Drawing for the job (mm, zero at the part's lowest x, y, z). A direction names the side the tool comes from. Give positions to 0.01 mm unless a question says otherwise; leave off trailing zeros. Loops run counter-clockwise (first coordinate to the right, second up) from the corner with the lowest first, then second, coordinate; pieces in that order, holes last. Notation, with made-up numbers: (53, 46.25) - (65, 46.25) arc R21 ccw to (65, 72.25) - close; hole circle Ø11 at (13.5, 16). An arc over 180 degrees is marked (long way). Return JSON: item names as keys, results as strings. Group by question number.
1) 3-axis set-ups, long thin cutter, end or side, ignore diameter. For the marked faces 4 and 5: which of +Z, -Z, +X, -X, +Y, -Y reach the whole face in a straight line?
2) Slice it at C-C (y = 11.5). List the corners of the cut face in (x, z), and give its area (4 significant figures).
3) Drill centre lines: probe 1 along Y at (x, z) = (23.7, 20); probe 2 along Z at (x, y) = (7.75, 26); probe 3 along X at (y, z) = (35.5, 35.5). Where is each one in solid material? Low to high. Write a range as from..to.
4) Drop flat-ended pins along their axis: pin 1 (8 mm diameter, centred on y = 20, z = 20, fed in from +X); pin 2 (6 mm diameter, centred on x = 14, y = 25.5, fed in from -Z); pin 3 (1 mm diameter, centred on x = 22, z = 6, fed in from -Y); pin 4 (12 mm diameter, centred on y = 22.5, z = 5, fed in from -X). Give the stop position or say it passes through.
5) Slice it at B-B (z = 35). List the corners of the cut face in (x, y).
6) Slice it at D-D (x = 14). List the corners of the cut face in (y, z), and give its area (3 significant figures).
7) Mould opens along Y. For the marked faces 1, 2 and 3 say: released by +Y, released by -Y, zero draft, split by the parting line, or undercut.
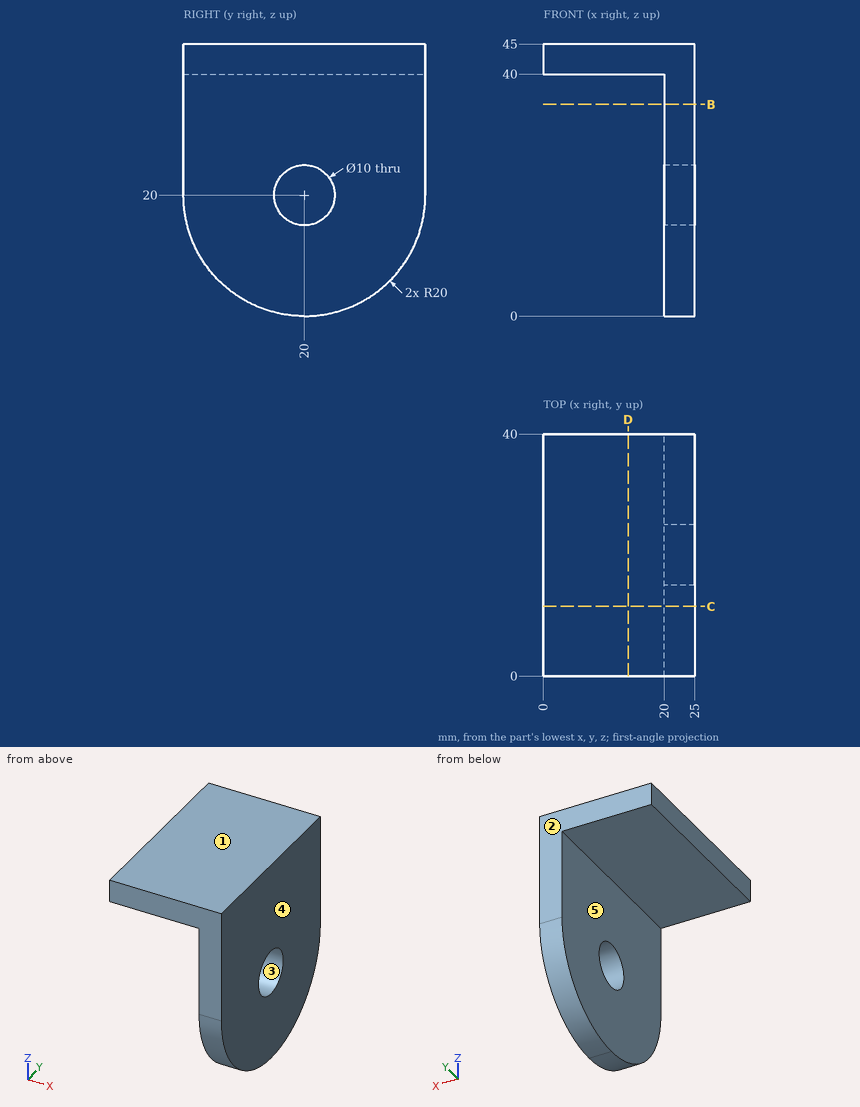
Results:
{
 "1": {"face 4": "+Z, -Z, +X, +Y, -Y", "face 5": "-Z, -X, +Y, -Y"},
 "2": {"outline": "(0, 40) - (20, 40) - (20, 1.9) - (25, 1.9) - (25, 45) - (0, 45) - close", "area": "315.5 mm2"},
 "3": {"probe 1": "0..15, 25..40", "probe 2": "40..45", "probe 3": "20..25"},
 "4": {"pin 1": "through", "pin 2": "z = 40", "pin 3": "y = 5.24", "pin 4": "x = 20"},
 "5": {"outline": "(20, 0) - (25, 0) - (25, 40) - (20, 40) - close"},
 "6": {"outline": "(0, 40) - (40, 40) - (40, 45) - (0, 45) - close", "area": "200 mm2"},
 "7": {"face 1": "zero draft", "face 2": "released by +Y", "face 3": "undercut"}
}
